```python
from build123d import *

# Parameters (mm, degrees)
F0_R     = 11.15
F1_DEPTH = 4
F3_DEPTH = 16.2
F4_R     = 11.15
F5_DEPTH = 1.5


with BuildPart() as f1:
    # F0 (on Top) → F1 (new body)
    with BuildSketch(Plane.XY):
        with BuildLine():
            ThreePointArc((-2.75, 14.7457621031), (-9.5851447563, -11.5379807592), (15, 0))
            ThreePointArc((15, 0), (11.5379807592, 9.5851447563), (2.75, 14.7457621031))
            Line((2.75, 14.7457621031), (4, 12.5806985936))
            Line((4, 12.5806985936), (0, 12.5806985936))
            Line((0, 12.5806985936), (-4, 12.5806985936))
            Line((-4, 12.5806985936), (-2.75, 14.7457621031))
        make_face()
        Circle(F0_R, mode=Mode.SUBTRACT)
        with BuildLine():
            Line((4, 12.5806985936), (2.75, 14.7457621031))
            ThreePointArc((2.75, 14.7457621031), (0, 15), (-2.75, 14.7457621031))
            Line((-2.75, 14.7457621031), (-4, 12.5806985936))
            Line((-4, 12.5806985936), (0, 12.5806985936))
            Line((0, 12.5806985936), (4, 12.5806985936))
        make_face()
    extrude(amount=F1_DEPTH)

    # F2 (on face) → F3 (cut)
    with BuildSketch(Plane.XY.offset(4)):
        with BuildLine():
            ThreePointArc((-11.3952045794, 9.7544509119), (-12.9903810568, 7.5), (-14.1452045794, 4.9913111911))
            Line((-14.1452045794, 4.9913111911), (-12.8952045794, 2.8262476817))
            Line((-12.8952045794, 2.8262476817), (-8.8952045794, 9.7544509119))
            Line((-8.8952045794, 9.7544509119), (-11.3952045794, 9.7544509119))
        make_face()
        with BuildLine():
            Line((-12.8952045794, -2.8262476817), (-14.1452045794, -4.9913111911))
            ThreePointArc((-14.1452045794, -4.9913111911), (-12.9903810568, -7.5), (-11.3952045794, -9.7544509119))
            Line((-11.3952045794, -9.7544509119), (-8.8952045794, -9.7544509119))
            Line((-8.8952045794, -9.7544509119), (-12.8952045794, -2.8262476817))
        make_face()
        with BuildLine():
            Line((-4, -12.5806985936), (-2.75, -14.7457621031))
            ThreePointArc((-2.75, -14.7457621031), (0, -15), (2.75, -14.7457621031))
            Line((2.75, -14.7457621031), (4, -12.5806985936))
            Line((4, -12.5806985936), (-4, -12.5806985936))
        make_face()
        with BuildLine():
            Line((8.8952045794, -9.7544509119), (11.3952045794, -9.7544509119))
            ThreePointArc((11.3952045794, -9.7544509119), (12.9903810568, -7.5), (14.1452045794, -4.9913111911))
            Line((14.1452045794, -4.9913111911), (12.8952045794, -2.8262476817))
            Line((12.8952045794, -2.8262476817), (8.8952045794, -9.7544509119))
        make_face()
        with BuildLine():
            ThreePointArc((14.1452045794, 4.9913111911), (12.9903810568, 7.5), (11.3952045794, 9.7544509119))
            Line((11.3952045794, 9.7544509119), (8.8952045794, 9.7544509119))
            Line((8.8952045794, 9.7544509119), (12.8952045794, 2.8262476817))
            Line((12.8952045794, 2.8262476817), (14.1452045794, 4.9913111911))
        make_face()
        with BuildLine():
            ThreePointArc((2.75, 14.7457621031), (0, 15), (-2.75, 14.7457621031))
            Line((-2.75, 14.7457621031), (-4, 12.5806985936))
            Line((-4, 12.5806985936), (4, 12.5806985936))
            Line((4, 12.5806985936), (2.75, 14.7457621031))
        make_face()
    extrude(amount=-F3_DEPTH, mode=Mode.SUBTRACT)

    # F4 (on face) → F5 (join)
    with BuildSketch(Plane(origin=(0, 0, 0), x_dir=(1, 0, 0), z_dir=(0, 0, -1))):
        with BuildLine():
            ThreePointArc((14.1452045794, -4.9913111911), (14.784756824, -2.5319884783), (15, 0))
            ThreePointArc((15, 0), (14.784756824, 2.5319884783), (14.1452045794, 4.9913111911))
            Line((14.1452045794, 4.9913111911), (12.8952045794, 2.8262476817))
            Line((12.8952045794, 2.8262476817), (8.8952045794, 9.7544509119))
            Line((8.8952045794, 9.7544509119), (11.3952045794, 9.7544509119))
            ThreePointArc((11.3952045794, 9.7544509119), (7.5, 12.9903810568), (2.75, 14.7457621031))
            Line((2.75, 14.7457621031), (4, 12.5806985936))
            Line((4, 12.5806985936), (-4, 12.5806985936))
            Line((-4, 12.5806985936), (-2.75, 14.7457621031))
            ThreePointArc((-2.75, 14.7457621031), (-7.5, 12.9903810568), (-11.3952045794, 9.7544509119))
            Line((-11.3952045794, 9.7544509119), (-8.8952045794, 9.7544509119))
            Line((-8.8952045794, 9.7544509119), (-12.8952045794, 2.8262476817))
            Line((-12.8952045794, 2.8262476817), (-14.1452045794, 4.9913111911))
            ThreePointArc((-14.1452045794, 4.9913111911), (-15, 0), (-14.1452045794, -4.9913111911))
            Line((-14.1452045794, -4.9913111911), (-12.8952045794, -2.8262476817))
            Line((-12.8952045794, -2.8262476817), (-8.8952045794, -9.7544509119))
            Line((-8.8952045794, -9.7544509119), (-11.3952045794, -9.7544509119))
            ThreePointArc((-11.3952045794, -9.7544509119), (-7.5, -12.9903810568), (-2.75, -14.7457621031))
            Line((-2.75, -14.7457621031), (-4, -12.5806985936))
            Line((-4, -12.5806985936), (4, -12.5806985936))
            Line((4, -12.5806985936), (2.75, -14.7457621031))
            ThreePointArc((2.75, -14.7457621031), (7.5, -12.9903810568), (11.3952045794, -9.7544509119))
            Line((11.3952045794, -9.7544509119), (8.8952045794, -9.7544509119))
            Line((8.8952045794, -9.7544509119), (12.8952045794, -2.8262476817))
            Line((12.8952045794, -2.8262476817), (14.1452045794, -4.9913111911))
        make_face()
        Circle(F4_R, mode=Mode.SUBTRACT)
        with BuildLine():
            Line((12.8952045794, 2.8262476817), (14.1452045794, 4.9913111911))
            ThreePointArc((14.1452045794, 4.9913111911), (12.9903810568, 7.5), (11.3952045794, 9.7544509119))
            Line((11.3952045794, 9.7544509119), (8.8952045794, 9.7544509119))
            Line((8.8952045794, 9.7544509119), (12.8952045794, 2.8262476817))
        make_face()
        with BuildLine():
            ThreePointArc((11.3952045794, -9.7544509119), (12.9903810568, -7.5), (14.1452045794, -4.9913111911))
            Line((14.1452045794, -4.9913111911), (12.8952045794, -2.8262476817))
            Line((12.8952045794, -2.8262476817), (8.8952045794, -9.7544509119))
            Line((8.8952045794, -9.7544509119), (11.3952045794, -9.7544509119))
        make_face()
        with BuildLine():
            Line((4, 12.5806985936), (2.75, 14.7457621031))
            ThreePointArc((2.75, 14.7457621031), (0, 15), (-2.75, 14.7457621031))
            Line((-2.75, 14.7457621031), (-4, 12.5806985936))
            Line((-4, 12.5806985936), (4, 12.5806985936))
        make_face()
        with BuildLine():
            ThreePointArc((-2.75, -14.7457621031), (0, -15), (2.75, -14.7457621031))
            Line((2.75, -14.7457621031), (4, -12.5806985936))
            Line((4, -12.5806985936), (-4, -12.5806985936))
            Line((-4, -12.5806985936), (-2.75, -14.7457621031))
        make_face()
        with BuildLine():
            Line((-8.8952045794, 9.7544509119), (-11.3952045794, 9.7544509119))
            ThreePointArc((-11.3952045794, 9.7544509119), (-12.9903810568, 7.5), (-14.1452045794, 4.9913111911))
            Line((-14.1452045794, 4.9913111911), (-12.8952045794, 2.8262476817))
            Line((-12.8952045794, 2.8262476817), (-8.8952045794, 9.7544509119))
        make_face()
        with BuildLine():
            ThreePointArc((-14.1452045794, -4.9913111911), (-12.9903810568, -7.5), (-11.3952045794, -9.7544509119))
            Line((-11.3952045794, -9.7544509119), (-8.8952045794, -9.7544509119))
            Line((-8.8952045794, -9.7544509119), (-12.8952045794, -2.8262476817))
            Line((-12.8952045794, -2.8262476817), (-14.1452045794, -4.9913111911))
        make_face()
    extrude(amount=F5_DEPTH)


solid = f1.part
```
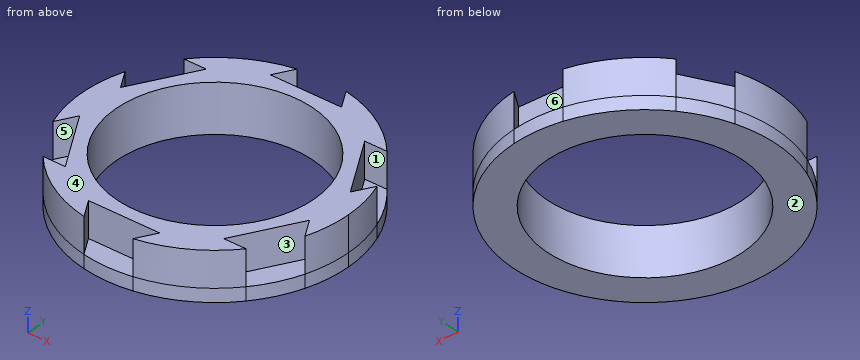
For this review, take the finished solid that the model builds, in its own axes (mm). Face numbers are marked on the shaded views. A direction names the side the tool comes from. Give positions to 0.01 mm unless a question says otherwise; leave off trailing zeros. Write each loop counter-clockwise with the first axis right and the second up, starting at its lowest first coordinate (ties: lowest second). Pieces come first, ordered by that corner, then holes.
Item 1: Take a section at D-D (x = -10.5). Give the boundary of the cut face in (y, z), and give its area (3 significant figures).
Item 2: Machinability: for the marked faces 1, 2 and 3, which of the approach directions +Z, -Z, +X, -X, +Y, -Y give a long, thin tool a straight path to every point of the face, cutting with its end or side? Answer none if there is none.
Item 3: Insertion check: P1, Ø2, axis at x = -1, z = 2.5, coming from the +Y side; P2, Ø1.2, axis at x = -10, z = 1.5, coming from the -Y side; P3, Ø2, axis at x = 10, z = 2.5, coming from the +Y side. Each pin has a flat end and moves straight along its axis. Give the tip position at first contact, or say it passes through.
Item 4: Take a section at B-B (x = 0). Give the boundary of the cut face in (y, z), and give its area (3 significant figures).
Item 5: Take a section at C-C (y = 8.5). Give the boundary of the cut face in (x, z), and give its area (3 significant figures).
Item 6: Wall thickness on probe 1 along Y at (x, z) = (0, 0.3); probe 2 along X at (y, z) = (0, -0.1): over which ranges is each line inside the solid? List them lowest first.
Item 7: Take a section at A-A (z = 2.25). Give the boundary of the cut face in (x, y), and give its area (3 significant figures).
Item 8: The part is to be moulded in two halves that separate along Y. For the marked faces 4, 5 and 6, say which applies: +Y half, -Y half, draft (parallel to the pull), parting line (faces both ways), or undercut.
Established:
1. outline: (-10.71, -1.5) - (-3.75, -1.5) - (-3.75, 4) - (-6.97, 4) - (-6.97, 0) - (-9.75, 0) - (-9.75, 4) - (-10.71, 4) - close; (3.75, -1.5) - (10.71, -1.5) - (10.71, 4) - (9.75, 4) - (9.75, 0) - (6.97, 0) - (6.97, 4) - (3.75, 4) - close
1. area: 54.3 mm2
2. face 1: +Z, +X
2. face 2: -Z, +X, -X, +Y, -Y
2. face 3: +Z
3. P1: stops at y = 12.58
3. P2: stops at y = -11.69
3. P3: stops at y = 12
4. outline: (-15, -1.5) - (-11.15, -1.5) - (-11.15, 4) - (-12.58, 4) - (-12.58, 0) - (-15, 0) - close; (11.15, -1.5) - (15, -1.5) - (15, 0) - (12.58, 0) - (12.58, 4) - (11.15, 4) - close
4. area: 23.0 mm2
5. outline: (-12.36, -1.5) - (-7.22, -1.5) - (-7.22, 4) - (-9.62, 4) - (-9.62, 0) - (-12.36, 0) - close; (7.22, -1.5) - (12.36, -1.5) - (12.36, 0) - (9.62, 0) - (9.62, 4) - (7.22, 4) - close
5. area: 34.7 mm2
6. probe 1: y = -12.58 to -11.15, 11.15 to 12.58
6. probe 2: x = -15 to -11.15, 11.15 to 15
7. outline: (-14.15, -4.99) - (-12.9, -2.83) - (-8.9, -9.75) - (-11.4, -9.75) arc R15 ccw to (-2.75, -14.75) - (-4, -12.58) - (4, -12.58) - (2.75, -14.75) arc R15 ccw to (11.4, -9.75) - (8.9, -9.75) - (12.9, -2.83) - (14.15, -4.99) arc R15 ccw to (14.15, 4.99) - (12.9, 2.83) - (8.9, 9.75) - (11.4, 9.75) arc R15 ccw to (2.75, 14.75) - (4, 12.58) - (-4, 12.58) - (-2.75, 14.75) arc R15 ccw to (-11.4, 9.75) - (-8.9, 9.75) - (-12.9, 2.83) - (-14.15, 4.99) arc R15 ccw to start; hole circle Ø22.3 at (0, 0)
7. area: 223 mm2
8. face 4: draft
8. face 5: -Y half
8. face 6: undercut
